Can you work these out from the model? Positions are in its coordinate system, mm. Face numbers are marked on the shaded views. Give positions to 0.01 mm unless a question says otherwise; leave off trailing zeros. Order: outer loops, then holes, each group sorted by start corner. A loop starts at its lowest first (then second) coordinate and runs counter-clockwise, first axis right, second up. Notation, with made-up numbers: (30.25, 21) - (34.25, 21) arc R19 ccw to (34.25, 35) - close; hole circle Ø7 at (61, -16.5). An arc over 180 degrees is marked (long way). Answer as a JSON object with one key per item and string values.
```python
from build123d import *

# Parameters (mm, degrees)
SKETCH1_R               = 38.1
BOSS_EXTRUDE1_DEPTH     = 4.445
SKETCH2_R               = 14.4145
SKETCH2_R_2             = 1.778
CUT_EXTRUDE1_DEPTH      = 1
CUT_EXTRUDE1_DEPTH_BACK = 5.445
CHAMFER1_SIZE           = 2.032
CHAMFER1_SIZE2          = 1.766390651
CHAMFER1_PART_2_SIZE    = 2.032
CHAMFER1_PART_2_SIZE2   = 1.766390651
SKETCH10_R              = 15.875
SKETCH10_R_2            = 6.35
BOSS_EXTRUDE5_DEPTH     = 7.62
CHAMFER2_SIZE           = 0.635


with BuildPart() as part:
    # Sketch1 → Boss-Extrude1 (new body)
    with BuildSketch(Plane(origin=(0, 0, 0), x_dir=(1, 0, 0), z_dir=(0, 1, 0))):
        Circle(SKETCH1_R)
    extrude(amount=BOSS_EXTRUDE1_DEPTH)

    # Sketch2 → Cut-Extrude1 (cut, two sides)
    with BuildSketch(Plane(origin=(0, 4.445, 0), x_dir=(1, 0, 0), z_dir=(0, 1, 0))) as cut_extrude1_sk:
        with Locations((-8.06, -14.01)):
            Circle(SKETCH2_R)
        with Locations((4.759999878, 30.270007278)):
            Circle(SKETCH2_R_2)
        with Locations((13.649999878, 27.730007278)):
            Circle(SKETCH2_R_2)
    extrude(amount=CUT_EXTRUDE1_DEPTH, mode=Mode.SUBTRACT)
    extrude(cut_extrude1_sk.sketch, amount=-CUT_EXTRUDE1_DEPTH_BACK, mode=Mode.SUBTRACT)

    # Chamfer1
    chamfer1_edges = [part.edges().sort_by_distance(p)[0] for p in [
        (2.981999878, 4.445, -30.270007278),
    ]]
    chamfer1_side = [part.faces().sort_by_distance(p)[0] for p in [
        (2.981999878, 2.2225, -30.270007278),
    ]]
    chamfer(chamfer1_edges, length=CHAMFER1_SIZE, length2=CHAMFER1_SIZE2, reference=chamfer1_side[0])

    # Chamfer1 part 2
    chamfer1_part_2_edges = [part.edges().sort_by_distance(p)[0] for p in [
        (11.871999878, 4.445, -27.730007278),
    ]]
    chamfer1_part_2_side = [part.faces().sort_by_distance(p)[0] for p in [
        (1.306244319, 4.445, -2.20411426),
    ]]
    chamfer(chamfer1_part_2_edges, length=CHAMFER1_PART_2_SIZE, length2=CHAMFER1_PART_2_SIZE2, reference=chamfer1_part_2_side[0])

    # Sketch10 → Boss-Extrude5 (add)
    with BuildSketch(Plane.XZ):
        with Locations((-8.06, 14.01)):
            Circle(SKETCH10_R)
        with Locations((-8.06, 14.01)):
            Circle(SKETCH10_R_2, mode=Mode.SUBTRACT)
    extrude(amount=-BOSS_EXTRUDE5_DEPTH)

    # Chamfer2
    chamfer2_edges = [part.edges().sort_by_distance(p)[0] for p in [
        (-14.41, 7.62, 14.01),
        (-14.41, 0, 14.01),
    ]]
    chamfer(chamfer2_edges, length=CHAMFER2_SIZE)


solid = part.part
```
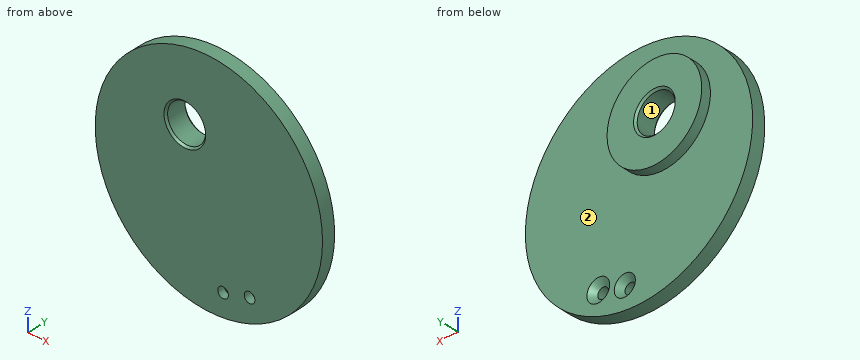
Q1. If we section it at C-C, the plane y = 6: Please give me the cut outline in (x, z) (3 decimals).
Recorded:
{"outline": "circle Ø31.75 at (-8.06, 14.01); hole circle Ø12.7 at (-8.06, 14.01)"}
Q2. I'm going to push flat-ended pins straight in: pin 1 Ø3 at (x, z) = (-25, -30) entering from +Y (3 decimals); pin 2 Ø4 at (y, z) = (1.5, 15) entering from +X; pin 3 Ø3 at (x, z) = (4.76, -30.27) entering from +Y. Where does each tip first touch, or does it pass through?
Recorded:
{"pin 1": "stops at y = 4.445", "pin 2": "stops at x = 35.81", "pin 3": "passes through"}
Q3. I need wall thicknesses on L1, parallel to Z at x = -8.06, y = 5.5 (3 decimals); L2, parallel to Y at x = -17, z = -24 (3 decimals); L3, parallel to Z at x = 4.76, y = 1.15. Which ranges of each line are inside material? Lowest first, please.
Recorded:
{"L1": "z = -1.865 to 7.66, 20.36 to 29.885", "L2": "y = 0 to 4.445", "L3": "z = -37.8 to -32.05, -28.49 to 37.8"}
Q4. We'd pull the mould along X, two halves only. Please class the marked faces 1 and 2: released by +X, released by -X, zero draft, split by the parting line, or undercut.
Recorded:
{"face 1": "undercut", "face 2": "zero draft"}
Q5. If we section it at D-D, the plane x = -20.5: Please give me the cut outline in (y, z) (3 decimals), then the cut area to 3 significant figures.
Recorded:
{"outline": "(0, -32.115) - (4.445, -32.115) - (4.445, 4.148) - (7.62, 4.148) - (7.62, 23.872) - (4.445, 23.872) - (4.445, 32.115) - (0, 32.115) - close", "area": "348 mm^2"}
Q6. If we section it at A-A, the plane x = 13.65: Please give me the cut outline in (y, z) (3 decimals), then the cut area to 3 significant figures.
Recorded:
{"outline": "(0, -35.571) - (4.445, -35.571) - (4.445, -31.54) - (2.679, -29.508) - (0, -29.508) - close; (0, -25.952) - (2.679, -25.952) - (4.445, -23.92) - (4.445, 35.571) - (0, 35.571) - close", "area": "297 mm^2"}
Q7. If we section it at B-B, the plane z = 14.01: Please give me the cut outline in (x, y) (3 decimals).
Recorded:
{"outline": "(-35.431, 0) - (-15.045, 0) - (-14.41, 0.635) - (-14.41, 6.985) - (-15.045, 7.62) - (-23.935, 7.62) - (-23.935, 4.445) - (-35.431, 4.445) - close; (-1.71, 0.635) - (-1.075, 0) - (35.431, 0) - (35.431, 4.445) - (7.815, 4.445) - (7.815, 7.62) - (-1.075, 7.62) - (-1.71, 6.985) - close"}
